For this review, use the dimensioned drawing (mm, ordinates from the lowest corner) and the shaded views. A direction names the side the tool comes from. Coordinates: 2 decimals unless noted, no trailing zeros. Loops run counter-clockwise (first coordinate to the right, second up) from the corner with the lowest first, then second, coordinate; pieces in that order, holes last. Notation, with made-up numbers: (53, -28) - (100, -28) arc R28 ccw to (100, 1) - close; hole circle Ø3 at (76.5, 41.5). An arc over 180 degrees is marked (long way). Answer in a Markdown table with one row per item. Add a question column.
(1) Mouldability with a two-part tool opening along X and no side actions: class the marked faces 4, 5, 6 and 7 as +X half, -X half, draft (parallel to the pull), parting line (faces both ways), or undercut.
(2) For P1, Ø10, axis at y = 15, z = 6, coming from the -X side; P2, Ø3, axis at x = 10.5, z = 9, coming from the +Y side; P3, Ø8, axis at y = 35, z = 4.5, coming from the -X side, all flat-tipped, find the tip position at first contact; note any pin that passes through.
(3) For line 1 along Y through (x, z) = (22.5, 2.75); line 2 along Y through (x, z) = (22.5, 17.75); line 3 along Y through (x, z) = (19.5, 6), list the stretches that pass through material, from the lowest coordinate up.
(4) We need section B-B on x = 22.5. Write out the cut boundary in (y, z), plus the area to 3 significant figures.
(5) We need section D-D on z = 9.25. Write out the cut boundary in (x, y).
(6) We need section C-C on y = 22.5. Write out the cut boundary in (x, z).
(7) Machinability: for the marked faces 1, 2 and 3, which of the approach directions +Z, -Z, +X, -X, +Y, -Y give a long, thin tool a straight path to every point of the face, cutting with its end or side? Answer none if there is none.
(8) We need section A-A on z = 5.25. Write out the cut boundary in (x, y), plus the area to 3 significant figures.
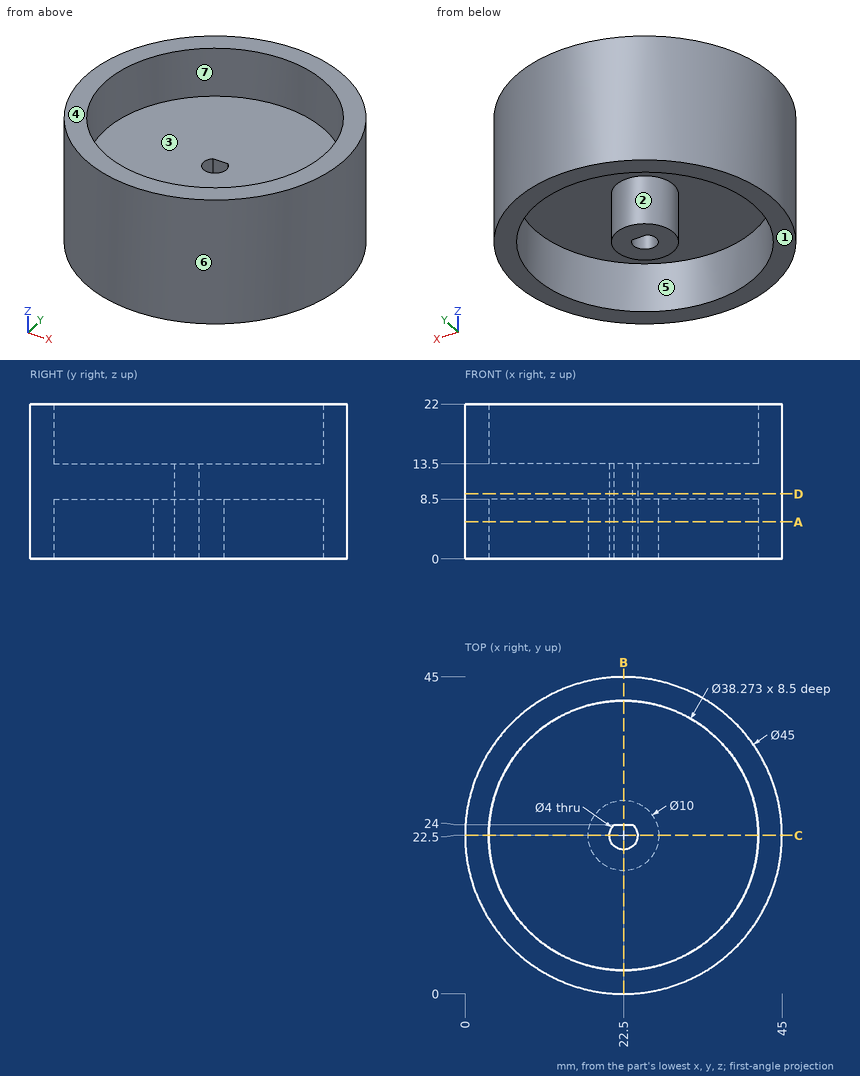
Outcome:
| question | item | result |
|---|---|---|
| 1 | face 4 | draft |
| 1 | face 5 | undercut |
| 1 | face 6 | parting line |
| 1 | face 7 | undercut |
| 2 | P1 | x = 0.14 |
| 2 | P2 | y = 42.4 |
| 2 | P3 | x = 1.67 |
| 3 | line 1 | 0 to 3.36, 17.5 to 20.5, 24 to 27.5, 41.64 to 45 |
| 3 | line 2 | 0 to 3.36, 41.64 to 45 |
| 3 | line 3 | 0.2 to 3.6, 18.5 to 26.5, 41.4 to 44.8 |
| 4 | outline | (0, 0) - (3.36, 0) - (3.36, 8.5) - (17.5, 8.5) - (17.5, 0) - (20.5, 0) - (20.5, 13.5) - (3.36, 13.5) - (3.36, 22) - (0, 22) - close; (24, 0) - (27.5, 0) - (27.5, 8.5) - (41.64, 8.5) - (41.64, 0) - (45, 0) - (45, 22) - (41.64, 22) - (41.64, 13.5) - (24, 13.5) - close |
| 4 | area | 377 mm² |
| 5 | outline | circle Ø45 at (22.5, 22.5); hole (21.18, 24) arc R2 ccw (long way) to (23.82, 24) - close |
| 6 | outline | (0, 0) - (3.36, 0) - (3.36, 8.5) - (17.5, 8.5) - (17.5, 0) - (20.5, 0) - (20.5, 13.5) - (3.36, 13.5) - (3.36, 22) - (0, 22) - close; (24.5, 0) - (27.5, 0) - (27.5, 8.5) - (41.64, 8.5) - (41.64, 0) - (45, 0) - (45, 22) - (41.64, 22) - (41.64, 13.5) - (24.5, 13.5) - close |
| 7 | face 1 | -Z, +X, -X, +Y, -Y |
| 7 | face 2 | -Z |
| 7 | face 3 | +Z |
| 8 | outline | circle Ø45 at (22.5, 22.5); circle Ø10 at (22.5, 22.5); hole circle Ø38.27 at (22.5, 22.5); hole (21.18, 24) arc R2 ccw (long way) to (23.82, 24) - close |
| 8 | area | 507 mm² |
